The model under review builds one solid part; all positions refer to its coordinate system, in mm. Face numbers are marked on the shaded views. A direction names the side the tool comes from. Round coordinates to 2 decimals unless told otherwise and drop trailing zeros. Order: outer loops, then holes, each group sorted by start corner. A loop starts at its lowest first (then second) coordinate and runs counter-clockwise, first axis right, second up. Notation, with made-up numbers: M 14.5,19 L 25.5,19 A22 cw 25.5,30 Z; hole C 10.5,72.25 d11. An arc over 180 degrees is marked long. Answer as a JSON object with one key per item and string values. Group by question number.
1) Insertion check: pin 1 Ø2.5 at (x, z) = (24.12, 41.79) entering from +Y; pin 2 Ø1 at (x, y) = (-36, 6.5) entering from +Z; pin 3 Ø5 at (y, z) = (33, -3.5) entering from +X. Each pin has a flat end and moves straight along its axis. Give the tip position at first contact, or say it passes through.
2) For the marked faces 1 and 2, list the 3-axis set-ups (+Z, -Z, +X, -X, +Y, -Y) from which the entire face can be reached by the end or side of a thin tool; tool diameter is ignored.
3) To check wall thickness, follow line 1 (Y direction, x = -2, z = 16); line 2 (X direction, y = 21, z = -3.5); line 3 (X direction, y = 20.5, z = -22). State the ranges of each line that lie inside material, in increasing order.
4) Consider section B-B, the plane y = 36.5. Write out the cut boundary in (x, z) (3 decimals), then the cut area to 3 significant figures.
5) Consider section A-A, the plane y = 22. Write out the cut boundary in (x, z).
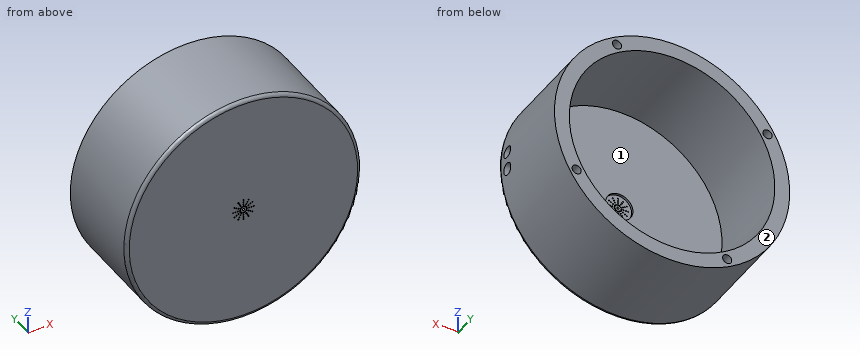
```python
from build123d import *

# Parameters (mm, degrees)
SKETCH1_R                = 51.5
BOSS_EXTRUDE1_DEPTH      = 42
SKETCH2_R                = 45
CUT_EXTRUDE1_DEPTH       = 40
FILLET1_R                = 1.5
SKETCH6_R                = 2
CUT_EXTRUDE6_DEPTH       = 10
CUT_EXTRUDE12_DEPTH      = 15
CUT_EXTRUDE12_DEPTH_BACK = 15
SKETCH15_R               = 2.6
SKETCH17_R               = 6
CUT_EXTRUDE13_DEPTH      = 1
SKETCH18_R               = 0.25
SKETCH18_R_2             = 0.5
CUT_EXTRUDE14_DEPTH      = 1


with BuildPart() as part:
    # Sketch1 → Boss-Extrude1 (new body)
    with BuildSketch(Plane(origin=(0, 0, 0), x_dir=(1, 0, 0), z_dir=(0, 1, 0))):
        with Locations(Location((0, 0, 0), (0, 0, 90))):
            Circle(SKETCH1_R)
    extrude(amount=BOSS_EXTRUDE1_DEPTH)

    # Sketch2 → Cut-Extrude1 (cut)
    with BuildSketch(Plane(origin=(0, 42, 0), x_dir=(1, 0, 0), z_dir=(0, 1, 0))):
        with Locations(Location((0, 0, 0), (0, 0, 270))):
            Circle(SKETCH2_R)
    extrude(amount=-CUT_EXTRUDE1_DEPTH, mode=Mode.SUBTRACT)

    # Fillet1
    fillet1_edges = [part.edges().sort_by_distance(p)[0] for p in [
        (0, 0, 51.5),
    ]]
    fillet(fillet1_edges, radius=FILLET1_R)

    # Sketch6 → Cut-Extrude6 (cut)
    with BuildSketch(Plane(origin=(0, 42, 0), x_dir=(1, 0, 0), z_dir=(0, 1, 0))):
        with Locations(Location((41.785725733, 24.125, 0), (0, 0, 270))):
            Circle(SKETCH6_R)
        with Locations(Location((-24.125, 41.785725733, 0), (0, 0, 270))):
            Circle(SKETCH6_R)
        with Locations(Location((24.125, -41.785725733, 0), (0, 0, 270))):
            Circle(SKETCH6_R)
        with Locations(Location((-41.785725733, -24.125, 0), (0, 0, 270))):
            Circle(SKETCH6_R)
    extrude(amount=-CUT_EXTRUDE6_DEPTH, mode=Mode.SUBTRACT)

    # Sketch15 → Cut-Extrude12 (cut, two sides: drawn at the far end of the back side and taken through both)
    with BuildSketch(Plane.ZY.offset(-47.5).offset(-CUT_EXTRUDE12_DEPTH_BACK)):
        with Locations((-4, 6)):
            Circle(SKETCH15_R)
        with Locations((4, 6)):
            Circle(SKETCH15_R)
    extrude(amount=CUT_EXTRUDE12_DEPTH + CUT_EXTRUDE12_DEPTH_BACK, mode=Mode.SUBTRACT)

    # Sketch17 → Cut-Extrude13 (cut)
    with BuildSketch(Plane(origin=(0, 2, 0), x_dir=(1, 0, 0), z_dir=(0, 1, 0))):
        with Locations(Location((0, 0, 0), (0, 0, 270))):
            Circle(SKETCH17_R)
    extrude(amount=-CUT_EXTRUDE13_DEPTH, mode=Mode.SUBTRACT)

    # Sketch18 → Cut-Extrude14 (cut)
    with BuildSketch(Plane(origin=(0, 1, 0), x_dir=(1, 0, 0), z_dir=(0, 1, 0))):
        with Locations(Location((-1.5, 0, 0), (0, 0, 270))):
            Circle(SKETCH18_R)
        with Locations(Location((-2.5, 0, 0), (0, 0, 270))):
            Circle(SKETCH18_R)
        with Locations(Location((-3.5, 0, 0), (0, 0, 270))):
            Circle(SKETCH18_R)
        with Locations(Location((-4.5, 0, 0), (0, 0, 270))):
            Circle(SKETCH18_R)
        with Locations(Location((-1.299038106, 0.75, 0), (0, 0, 270))):
            Circle(SKETCH18_R)
        with Locations(Location((-2.165063509, 1.25, 0), (0, 0, 270))):
            Circle(SKETCH18_R)
        with Locations(Location((-3.031088913, 1.75, 0), (0, 0, 270))):
            Circle(SKETCH18_R)
        with Locations(Location((-3.897114317, 2.25, 0), (0, 0, 270))):
            Circle(SKETCH18_R)
        with Locations(Location((-0.75, 1.299038106, 0), (0, 0, 270))):
            Circle(SKETCH18_R)
        with Locations(Location((-1.25, 2.165063509, 0), (0, 0, 270))):
            Circle(SKETCH18_R)
        with Locations(Location((-1.75, 3.031088913, 0), (0, 0, 270))):
            Circle(SKETCH18_R)
        with Locations(Location((-2.25, 3.897114317, 0), (0, 0, 270))):
            Circle(SKETCH18_R)
        with Locations(Location((0, 4.5, 0), (0, 0, 270))):
            Circle(SKETCH18_R)
        with Locations(Location((0, 3.5, 0), (0, 0, 270))):
            Circle(SKETCH18_R)
        with Locations(Location((0, 2.5, 0), (0, 0, 270))):
            Circle(SKETCH18_R)
        with Locations(Location((0, 1.5, 0), (0, 0, 270))):
            Circle(SKETCH18_R)
        with Locations(Location((0.75, 1.299038106, 0), (0, 0, 270))):
            Circle(SKETCH18_R)
        with Locations(Location((1.25, 2.165063509, 0), (0, 0, 270))):
            Circle(SKETCH18_R)
        with Locations(Location((1.75, 3.031088913, 0), (0, 0, 270))):
            Circle(SKETCH18_R)
        with Locations(Location((2.25, 3.897114317, 0), (0, 0, 270))):
            Circle(SKETCH18_R)
        with Locations(Location((3.897114317, 2.25, 0), (0, 0, 270))):
            Circle(SKETCH18_R)
        with Locations(Location((3.031088913, 1.75, 0), (0, 0, 270))):
            Circle(SKETCH18_R)
        with Locations(Location((2.165063509, 1.25, 0), (0, 0, 270))):
            Circle(SKETCH18_R)
        with Locations(Location((1.299038106, 0.75, 0), (0, 0, 270))):
            Circle(SKETCH18_R)
        with Locations(Location((4.5, 0, 0), (0, 0, 270))):
            Circle(SKETCH18_R)
        with Locations(Location((3.5, 0, 0), (0, 0, 270))):
            Circle(SKETCH18_R)
        with Locations(Location((2.5, 0, 0), (0, 0, 270))):
            Circle(SKETCH18_R)
        with Locations(Location((1.5, 0, 0), (0, 0, 270))):
            Circle(SKETCH18_R)
        with Locations(Location((3.897114317, -2.25, 0), (0, 0, 270))):
            Circle(SKETCH18_R)
        with Locations(Location((3.031088913, -1.75, 0), (0, 0, 270))):
            Circle(SKETCH18_R)
        with Locations(Location((2.165063509, -1.25, 0), (0, 0, 270))):
            Circle(SKETCH18_R)
        with Locations(Location((1.299038106, -0.75, 0), (0, 0, 270))):
            Circle(SKETCH18_R)
        with Locations(Location((2.25, -3.897114317, 0), (0, 0, 270))):
            Circle(SKETCH18_R)
        with Locations(Location((1.75, -3.031088913, 0), (0, 0, 270))):
            Circle(SKETCH18_R)
        with Locations(Location((1.25, -2.165063509, 0), (0, 0, 270))):
            Circle(SKETCH18_R)
        with Locations(Location((0.75, -1.299038106, 0), (0, 0, 270))):
            Circle(SKETCH18_R)
        with Locations(Location((0, -1.6, 0), (0, 0, 270))):
            Circle(SKETCH18_R)
        with Locations(Location((0, -2.5, 0), (0, 0, 270))):
            Circle(SKETCH18_R)
        with Locations(Location((0, -3.5, 0), (0, 0, 270))):
            Circle(SKETCH18_R)
        with Locations(Location((0, -4.5, 0), (0, 0, 270))):
            Circle(SKETCH18_R)
        with Locations(Location((-0.75, -1.299038106, 0), (0, 0, 270))):
            Circle(SKETCH18_R)
        with Locations(Location((-1.25, -2.165063509, 0), (0, 0, 270))):
            Circle(SKETCH18_R)
        with Locations(Location((-1.75, -3.031088913, 0), (0, 0, 270))):
            Circle(SKETCH18_R)
        with Locations(Location((-2.25, -3.897114317, 0), (0, 0, 270))):
            Circle(SKETCH18_R)
        with Locations(Location((-1.299038106, -0.75, 0), (0, 0, 270))):
            Circle(SKETCH18_R)
        with Locations(Location((-2.165063509, -1.25, 0), (0, 0, 270))):
            Circle(SKETCH18_R)
        with Locations(Location((-3.031088913, -1.75, 0), (0, 0, 270))):
            Circle(SKETCH18_R)
        with Locations(Location((-3.897114317, -2.25, 0), (0, 0, 270))):
            Circle(SKETCH18_R)
        with Locations(Location((0, 0, 0), (0, 0, 270))):
            Circle(SKETCH18_R_2)
    extrude(amount=-CUT_EXTRUDE14_DEPTH, mode=Mode.SUBTRACT)


solid = part.part
```
Results list:
{
 "1": {"pin 1": "y = 32", "pin 2": "z = 37.31", "pin 3": "x = 51.49"},
 "2": {"face 1": "+Y", "face 2": "+Z, -Z, +X, -X, +Y"},
 "3": {"line 1": "0 to 2", "line 2": "-51.38 to -44.86, 44.86 to 51.38", "line 3": "-46.56 to -39.26, 39.26 to 46.56"},
 "4": {"outline": "C 0,0 d103; hole C 0,0 d90; hole C -41.786,24.125 d4; hole C -24.125,-41.786 d4; hole C 24.125,41.786 d4; hole C 41.786,-24.125 d4", "area": "1,920 mm^2"},
 "5": {"outline": "C 0,0 d103; hole C 0,0 d90"}
}
